```python
from build123d import *

# Parameters (mm, degrees)
CYLINDER007_R     = 4
CYLINDER007_DEPTH = 100
CYLINDER013_R     = 7.5
CYLINDER013_DEPTH = 24


with BuildPart() as rod_cylinder:
    # Cylinder007 → Cylinder007 (new body)
    with BuildSketch(Plane(origin=(42, 0, -122), x_dir=(1, 0, 0), z_dir=(0, 0, 1))):
        Circle(CYLINDER007_R)
    extrude(amount=CYLINDER007_DEPTH)


with BuildPart() as rod_fusion:
    # Cylinder013 → Cylinder013 (new body)
    with BuildSketch(Plane(origin=(42, 0, -91), x_dir=(1, 0, 0), z_dir=(0, 0, 1))):
        Circle(CYLINDER013_R)
    extrude(amount=CYLINDER013_DEPTH)

    # Fusion005: union rod cylinder
    add(rod_cylinder.part)


solid = rod_fusion.part
```
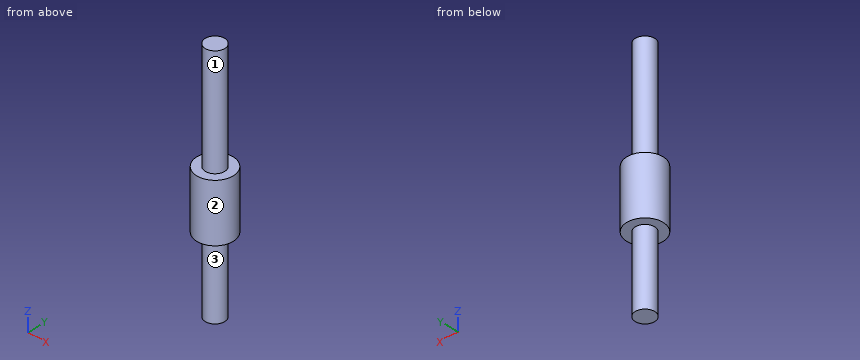
Work out the finished part from the listing and answer in its coordinate system (mm). Face numbers are marked on the shaded views. A direction names the side the tool comes from. Round coordinates to 2 decimals unless told otherwise and drop trailing zeros. Write each loop counter-clockwise with the first axis right and the second up, starting at its lowest first coordinate (ties: lowest second). Pieces come first, ordered by that corner, then holes. Notation, with made-up numbers: (0.5, -24) - (7.5, -24) arc R28 ccw to (7.5, 9) - close; hole circle Ø9 at (54.5, 70). An arc over 180 degrees is marked (long way). Return JSON: item names as keys, results as strings. Group by question number.
Q1. Find the intervals of material crossed by L1, parallel to Z at x = 38.5, y = 2.25; L2, parallel to X at y = 0.25, z = -27; L3, parallel to Y at x = 39.75, z = -40, in increasing order.
Q2. The part is cut by section A-A on y = 0. Write down the section's boundary in (x, z), then the cut area to 3 significant figures.
Q3. The part is cut by section D-D on z = -31. Write down the section's boundary in (x, y).
Q4. The part is cut by section B-B on x = 42. Write down the section's boundary in (y, z), then the cut area to 3 significant figures.
Q5. Each of these flat-tipped pins is pushed along its axis until it touches: pin 1 Ø5 at (y, z) = (-2.5, -52) entering from +X; pin 2 Ø1.5 at (x, y) = (38, -5) entering from -Z; pin 3 Ø1 at (x, y) = (36.5, -1.5) entering from +Z. Where does it stop, or does it pass through?
Q6. For the marked faces 1, 2 and 3, determine the directions among +Z, -Z, +X, -X, +Y, -Y from which every point of the face is accessible in a straight line to the end or side of a thin tool.
Q7. The part is cut by section C-C on z = -83.5. Write down the section's boundary in (x, y).
Solved:
{
 "1": {"L1": "-91 to -67", "L2": "38.01 to 45.99", "L3": "-3.31 to 3.31"},
 "2": {"outline": "(34.5, -91) - (38, -91) - (38, -122) - (46, -122) - (46, -91) - (49.5, -91) - (49.5, -67) - (46, -67) - (46, -22) - (38, -22) - (38, -67) - (34.5, -67) - close", "area": "968 mm²"},
 "3": {"outline": "circle Ø8 at (42, 0)"},
 "4": {"outline": "(-7.5, -91) - (-4, -91) - (-4, -122) - (4, -122) - (4, -91) - (7.5, -91) - (7.5, -67) - (4, -67) - (4, -22) - (-4, -22) - (-4, -67) - (-7.5, -67) - close", "area": "968 mm²"},
 "5": {"pin 1": "x = 46", "pin 2": "z = -91", "pin 3": "z = -67"},
 "6": {"face 1": "+Z", "face 2": "+Z, -Z", "face 3": "-Z"},
 "7": {"outline": "circle Ø15 at (42, 0)"}
}
